```python
from build123d import *

# Parameters (mm, degrees)
BOSS_EXTRUDE1_DEPTH     = 300
CUT_EXTRUDE1_DEPTH      = 856.862138431
CUT_EXTRUDE1_DEPTH_BACK = 856.862138431
SKETCH2_R               = 7.5


with BuildPart() as part:
    # Sketch1 → Boss-Extrude1 (new body)
    with BuildSketch(Plane(origin=(0, 0, 0), x_dir=(0, 0, -1), z_dir=(1, 0, 0))):
        Polygon((-400, 0), (400, 0), (400, -50), (385, -50), (385, -25), (375, -25), (375, -50), (360, -50), (360, -25), (-360, -25), (-360, -50), (-375, -50), (-375, -25), (-385, -25), (-385, -50), (-400, -50), align=None)
    extrude(amount=BOSS_EXTRUDE1_DEPTH)

    # Sketch2 → Cut-Extrude1 (cut, two sides: drawn at the far end of the back side and taken through both)
    with BuildSketch(Plane.XY.offset(400).offset(-CUT_EXTRUDE1_DEPTH_BACK)):
        with Locations((50, -37.5)):
            Circle(SKETCH2_R)
        with Locations((250, -37.5)):
            Circle(SKETCH2_R)
    extrude(amount=CUT_EXTRUDE1_DEPTH + CUT_EXTRUDE1_DEPTH_BACK, mode=Mode.SUBTRACT)


solid = part.part
```
Can you work these out from the model? Positions are in its coordinate system, mm. A direction names the side the tool comes from. Give positions to 0.01 mm unless a question says otherwise; leave off trailing zeros. Loops run counter-clockwise (first coordinate to the right, second up) from the corner with the lowest first, then second, coordinate; pieces in that order, holes last. Notation, with made-up numbers: M 44.5,-16.75 L 77.5,-16.75 A11 cw 77.5,-12.75 Z; hole C -11.75,33 d3. An arc over 180 degrees is marked long. One line per question, with ' | ' between items. Start each with the question number.
Q1. If we section it at A-A (x = 50): State how many separate pieces and enclosed holes the cut face has, plus the area to 3 significant figures.
Q2. For faces 1 (the flat face through (148, -38, -360)), 2 (the cylindrical face through (53.461, -44.154, -392.605)), which set-ups out of +Z, -Z, +X, -X, +Y, -Y let a thin tool reach every point of the face, with its end or its side?
Q3. If we section it at B-B (x = 147): Please give me the cut outline in (y, z), plus the area to 3 significant figures.
Q4. If we mould it in two halves opening along Y, with no side actions, what happens to faces 3 (the flat face through (148, -25, -5)), 4 (the cylindrical face through (256.93, -40.37, 367.4)), 5 (the flat face through (148, 0, 6))? For each: +Y half, -Y half, draft (parallel to the pull), parting line (faces both ways), or undercut.
Q5. If I drill on line 1 (X direction, y = -37.5, z = 394); line 2 (Z direction, x = 113, y = -43); line 3 (Y direction, x = 50, z = 368), over which ranges is the centre line in solid material (lowest first)? Write a range as from..to.
Q6. For pin 1 Ø10 at (x, z) = (97.5, -196) entering from +Y; pin 2 Ø13.5 at (x, y) = (50, -37.5) entering from -Z; pin 3 Ø1 at (x, z) = (88, -64) entering from -Y, each with a flat end and sliding along its axis, tell me the tip position at first contact or that it passes through.
Q7. If we section it at D-D (z = 27): Please give me the cut outline in (x, y), plus the area to 3 significant figures.
Computed:
1) separate pieces: 5 | enclosed holes: 0 | area: 20,600 mm²
2) face 1: +X, -X, -Y | face 2: +Z, -Z
3) outline: M -50,-400 L 0,-400 L 0,400 L -50,400 L -50,385 L -25,385 L -25,375 L -50,375 L -50,360 L -25,360 L -25,-360 L -50,-360 L -50,-375 L -25,-375 L -25,-385 L -50,-385 Z | area: 21,500 mm²
4) face 3: -Y half | face 4: undercut | face 5: +Y half
5) line 1: x = 0..42.5, 57.5..242.5, 257.5..300 | line 2: z = -400..-385, -375..-360, 360..375, 385..400 | line 3: y = -50..-45, -30..0
6) pin 1: stops at y = 0 | pin 2: passes through | pin 3: stops at y = -25
7) outline: M 0,-25 L 300,-25 L 300,0 L 0,0 Z | area: 7,500 mm²
